```python
from build123d import *

# Parameters (mm, degrees)
F1_DEPTH        = 69.85
F3_DEPTH        = 1.27
F3_TAPER        = 3
F4_T            = 6.35
F4_T3_DEPTH     = 60.96
F4_T5_DEPTH     = 60.96
F4_T7_DEPTH     = 60.96
F4_T10_ANGLE    = 90.000000001
F4_T12_ANGLE    = 90.000000001
F4_T14_ANGLE    = 90.000000001
F4_T16_ANGLE    = 90.000000001
F6_DEPTH        = 6.35
F8_D            = 2.54
F8_DEPTH        = 12.7
F8_TIP          = 0.7630929862
F7_R            = 15.24
F9_DEPTH        = 6.3499999999
F11_D           = 3.302
F11_DEPTH       = 12.7
F11_CBORE_D     = 6.35
F11_CBORE_DEPTH = 1.27
F11_TIP         = 0.992020882
F13_ANGLE       = 180


# Not quite as in the source:
# - a shell that OpenCascade refuses in one call is made with other operations: the cavity is built on its own and cut out


with BuildPart() as f1:
    # F0 (on Top) → F1 (new body)
    with BuildSketch(Plane.XY):
        Polygon((0, 63.5), (0, 0), (17.4534594442, -17.4534594442), (53.5082043519, 18.6012854634), align=None)
    extrude(amount=-F1_DEPTH)

    # F2 (on face) → F3 (cut)
    with BuildSketch(Plane(origin=(31.2676461581, 37.2633296409, 0), x_dir=(-0.7660444431, 0.6427876097, 0), z_dir=(0.6427876097, 0.7660444431, 0))):
        with BuildLine():
            ThreePointArc((-24.5879867849, -59.055), (-22.7281148454, -63.5451280605), (-18.2379867849, -65.405))
            Line((-18.2379867849, -65.405), (30.0220132151, -65.405))
            ThreePointArc((30.0220132151, -65.405), (34.5121412756, -63.5451280605), (36.3720132151, -59.055))
            Line((36.3720132151, -59.055), (36.3720132151, -10.795))
            ThreePointArc((36.3720132151, -10.795), (34.5121412756, -6.3048719395), (30.0220132151, -4.445))
            Line((30.0220132151, -4.445), (-18.2379867849, -4.445))
            ThreePointArc((-18.2379867849, -4.445), (-22.7281148454, -6.3048719395), (-24.5879867849, -10.795))
            Line((-24.5879867849, -10.795), (-24.5879867849, -59.055))
        make_face()
    extrude(amount=-F3_DEPTH, taper=F3_TAPER, mode=Mode.SUBTRACT)

    # F4: shell of thickness 6.35, made by hand


with BuildPart() as f4_core1:
    # F4_t2: copy of F1
    add(f1.part)

    # the walls: a layer under each face that stays
    f4_faces = [f4_core1.faces().sort_by_distance(p)[0] for p in [
        (49.6861897553, 21.8083365017, -64.8607142857),
        (35.480831898, 0.5739130096, -34.925),
        (26.7541021759, 23.0232702779, 0),
        (0, 31.75, -34.925),
        (48.2521957288, 22.1826667317, -63.5215962965),
        (26.3459320438, 40.5642045103, -65.3717210602),
        (4.4396683587, 58.9457422889, -63.5215962965),
        (3.0223905645, 60.1349795634, -34.925),
        (4.4396683587, 58.9457422889, -6.3284037035),
        (26.3459320438, 40.5642045103, -4.4782789398),
        (48.2521957288, 22.1826667317, -6.3284037035),
        (49.6694735231, 20.9934294573, -34.925),
        (8.7267297221, -8.7267297221, -34.925),
        (25.9377619116, 40.0777662889, -34.925),
    ]]
    thicken(f4_faces, amount=-F4_T, mode=Mode.SUBTRACT)

    # F4_s4 → F4_t3 (cut)
    with BuildSketch(Plane(origin=(18.8354906441, -15.8048532525, 0), x_dir=(0, 0, 1), z_dir=(-0.7660444431, 0.6427876097, 0))):
        Polygon((-65.2750291449, 47.4406454713), (-71.679739666, 47.0414888159), (-71.3643671189, 41.0238221381), (-65.3384421203, 41.0238221381), align=None)
    extrude(amount=F4_T3_DEPTH, mode=Mode.SUBTRACT)

    # F4_s6 → F4_t5 (cut)
    with BuildSketch(Plane.XY.offset(-65.405)):
        Polygon((2.7312439473, 59.63757862), (-2.4316219096, 63.4486754488), (-6.0581141021, 58.636157764), (-1.4419877423, 54.762767838), align=None)
        Polygon((49.2301862972, 20.6203332441), (53.8799062493, 16.1976929397), (49.7702352824, 11.7906103863), (45.1541089225, 15.6640003123), align=None)
    extrude(amount=F4_T5_DEPTH, mode=Mode.SUBTRACT)

    # F4_s8 → F4_t7 (cut)
    with BuildSketch(Plane(origin=(-27.8625786085, 23.379479434, 0), x_dir=(0, 0, 1), z_dir=(0.7660444431, -0.6427876097, 0))):
        Polygon((-4.5749708551, -47.4406454713), (1.829739666, -47.0414888159), (1.514367119, -41.0238221381), (-4.5115578797, -41.0238221381), align=None)
    extrude(amount=F4_T7_DEPTH, mode=Mode.SUBTRACT)

    # F4_s9 → F4_t10 (revolve, cut)
    with BuildSketch(Plane.XY.offset(-59.055)):
        Polygon((49.2301862972, 20.6203332441), (53.8799062493, 16.1976929397), (49.7702352824, 11.7906103863), (45.1541089225, 15.6640003123), align=None)
    revolve(axis=Axis((44.4224143241, 24.5673012672, -59.055), (0.6427876097, 0.7660444431, 0)), revolution_arc=F4_T10_ANGLE, mode=Mode.SUBTRACT)

    # F4_s11 → F4_t12 (revolve, cut)
    with BuildSketch(Plane(origin=(-22.9981963947, 19.2977781125, 0), x_dir=(0, 0, 1), z_dir=(0.7660444431, -0.6427876097, 0))):
        Polygon((-65.2750291449, -47.4406454713), (-71.679739666, -47.0414888159), (-71.364367119, -41.0238221381), (-65.3384421203, -41.0238221381), align=None)
    revolve(axis=Axis((7.4531094992, 55.5882313107, -59.055), (0.6427876097, 0.7660444431, 0)), revolution_arc=F4_T12_ANGLE, mode=Mode.SUBTRACT)

    # F4_s13 → F4_t14 (revolve, cut)
    with BuildSketch(Plane.XY.offset(-10.795)):
        Polygon((2.7312439473, 59.63757862), (-2.4316219096, 63.4486754488), (-6.0581141021, 58.636157764), (-1.4419877423, 54.762767838), align=None)
    revolve(axis=Axis((7.4531094992, 55.5882313107, -10.795), (0.6427876097, 0.7660444431, 0)), revolution_arc=F4_T14_ANGLE, mode=Mode.SUBTRACT)

    # F4_s15 → F4_t16 (revolve, cut)
    with BuildSketch(Plane(origin=(13.9711084303, -11.723151931, 0), x_dir=(0, 0, 1), z_dir=(-0.7660444431, 0.6427876097, 0))):
        Polygon((-4.5749708551, 47.4406454713), (1.829739666, 47.0414888159), (1.514367119, 41.0238221381), (-4.5115578797, 41.0238221381), align=None)
    revolve(axis=Axis((44.4224143241, 24.5673012672, -10.795), (0.6427876097, 0.7660444431, 0)), revolution_arc=F4_T16_ANGLE, mode=Mode.SUBTRACT)


with BuildPart() as f1_1:
    add(f1.part)

    # what is left inside the walls is the cavity
    f4_cavity = [f4_core1.part.solids().sort_by_distance(p)[0] for p in [
        (24.742436, 32.708534, -27.516667),
    ]]
    add(f4_cavity, mode=Mode.SUBTRACT)

    # F5 (on face) → F6 (cut, through all)
    with BuildSketch(Plane(origin=(17.4534594442, -17.4534594442, 0), x_dir=(0.7071067812, 0.7071067812, 0), z_dir=(0.7071067812, -0.7071067812, 0))):
        with BuildLine():
            Line((44.6391092363, -6.35), (6.35, -6.35))
            Line((6.35, -6.35), (6.35, -26.6769132179))
            ThreePointArc((6.35, -26.6769132179), (11.4220747655, -47.42814024), (25.4945546181, -63.5))
            ThreePointArc((25.4945546181, -63.5), (39.5670344708, -47.42814024), (44.6391092363, -26.6769132179))
            Line((44.6391092363, -26.6769132179), (44.6391092363, -6.35))
        make_face()
    extrude(amount=-F6_DEPTH, mode=Mode.SUBTRACT)

    # F8
    with Locations(Plane(origin=(30.4513058938, 36.2904531982, 0), x_dir=(-0.7660444431, 0.6427876097, 0), z_dir=(0.6427876097, 0.7660444431, 0))):
        with Locations((27.4820132151, -34.925), (-15.6979867849, -34.925)):
            Hole(F8_D / 2, depth=F8_DEPTH)
            with Locations((0, 0, -(F8_DEPTH + F8_TIP / 2))):  # 118° drill point
                Cone(0, F8_D / 2, F8_TIP, mode=Mode.SUBTRACT)

    # F7 (on face) → F9 (cut, through all)
    with BuildSketch(Plane(origin=(30.4513058938, 36.2904531982, 0), x_dir=(-0.7660444431, 0.6427876097, 0), z_dir=(0.6427876097, 0.7660444431, 0))):
        with Locations((5.8920132151, -34.925)):
            Circle(F7_R)
    extrude(amount=-F9_DEPTH, mode=Mode.SUBTRACT)

    # F11
    with Locations(Plane.YZ.offset(6.35)):
        with Locations((34.9977662889, -34.925)):
            CounterBoreHole(F11_D / 2, F11_CBORE_D / 2, F11_CBORE_DEPTH, depth=F11_DEPTH)
            with Locations((0, 0, -(F11_DEPTH + F11_TIP / 2))):  # 118° drill point
                Cone(0, F11_D / 2, F11_TIP, mode=Mode.SUBTRACT)

    # F12: F1 across face


with BuildPart() as f1_2:
    add(f1_1.part)
    add(f1_1.part.mirror(Plane(origin=(8.7267297221, -8.7267297221, -34.925), x_dir=(0.7071067812, -0.7071067812, 0), z_dir=(-0.7071067812, -0.7071067812, 0))))


with BuildPart() as f1_3:
    # F13: moved
    add(f1_2.part.rotate(Axis((-31.75, 0, 0), (-1, 0, 0)), F13_ANGLE))


solid = f1_3.part
```
Read the model definition and answer for the solid it produces. Units are mm, in the model's axes. A direction names the side the tool comes from. Give positions to 0.01 mm unless a question says otherwise; leave off trailing zeros. One line per item, written item: value. Start each with the question number.
(1) Straight lines are drawn through the part: L1, parallel to Y at x = -35.5, z = 56.5; L2, parallel to Y at x = 11, z = 48; L3, parallel to X at y = -14.5, z = 13.5. For each, find the intervals that lie inside material, in ascending order.
(2) For a pull along X with two mould halves and no side action, classify faces 5 (the conical face through (-22.14, 48.28, 63.47)), 6 (the flat face through (27.129, -40.736, 3.392)), 7 (the cylindrical face through (7.26, 23.22, 47.16)), 8 (the flat face through (3, 3, 0)) as released by +X, released by -X, zero draft, split by the parting line, or undercut.
(3) Flat-ended cylindrical pins translate along their axes: P1, Ø1.5, axis at y = -13, z = 61, coming from the +X side; P2, Ø4, axis at y = 13, z = 45, coming from the -X side; P3, Ø10, axis at x = -35, z = 34.92, coming from the +Y side; P4, Ø2, axis at x = -35, z = 34.92, coming from the -Y side. Find the tip coordinate at first contact, or state that the pin passes through.
(4) A tool of negligible diameter and unlimited length cuts with its end or side. For faces 1 (the conical face through (4.397, -58.97, 6.378)), 2 (the cylindrical face through (-37.93, 5.72, 36.14)), 3 (the flat face through (12.305, 3.325, 37.656)), 4 (the flat face through (27.292, -1.365, 62.352)), from which of +Z, -Z, +X, -X, +Y, -Y can it reach the whole face along a straight path? Write none if from no direction.
(5) The part is cut by section A-A (x = 29). State how many separate pieces and enclosed holes the cut face has, and give its area (3 significant figures).
Taken from the geometry:
1. L1: 0 to 6.35, 21.51 to 31.39
1. L2: -52.61 to -44.32, 2.02 to 23.91
1. L3: 0 to 6.35, 48.63 to 49.41
2. face 5: released by -X
2. face 6: released by +X
2. face 7: undercut
2. face 8: zero draft
3. P1: x = 48.66
3. P2: x = -52.61
3. P3: y = 37.95
3. P4: through
4. face 1: +X
4. face 2: +Y
4. face 3: none
4. face 4: +Z
5. separate pieces: 3
5. enclosed holes: 0
5. area: 695 mm^2
